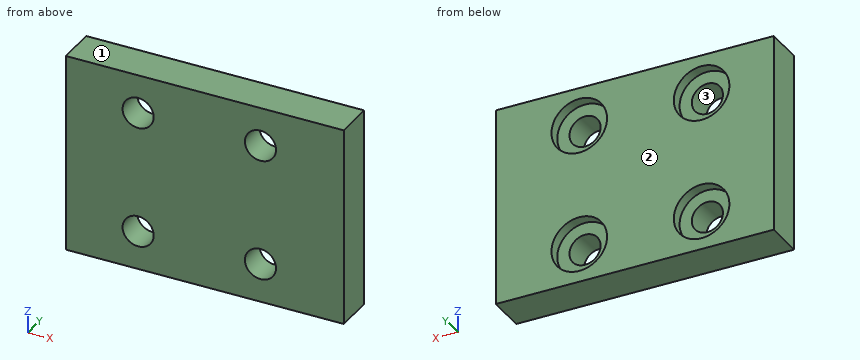
```python
from build123d import *

# Parameters (mm, degrees)
SKETCH1_W           = 50
SKETCH1_H           = 36
BOSS_EXTRUDE1_DEPTH = 7
SKETCH2_R           = 2.8
CUT_EXTRUDE1_DEPTH  = 63.008063992
SKETCH3_R           = 5
CUT_EXTRUDE2_DEPTH  = 2


with BuildPart() as part:
    # Sketch1 → Boss-Extrude1 (new body)
    with BuildSketch(Plane(origin=(0, 0, 0), x_dir=(1, 0, 0), z_dir=(0, 1, 0))):
        with Locations((25, 18)):
            Rectangle(SKETCH1_W, SKETCH1_H)
    extrude(amount=BOSS_EXTRUDE1_DEPTH)

    # Sketch2 → Cut-Extrude1 (cut, through all)
    with BuildSketch(Plane(origin=(0, 7, 0), x_dir=(1, 0, 0), z_dir=(0, 1, 0))):
        with Locations(Location((13, 29, 0), (0, 0, 270))):
            Circle(SKETCH2_R)
        with Locations(Location((13, 7, 0), (0, 0, 90))):
            Circle(SKETCH2_R)
        with Locations(Location((35, 29, 0), (0, 0, 270))):
            Circle(SKETCH2_R)
        with Locations(Location((35, 7, 0), (0, 0, 270))):
            Circle(SKETCH2_R)
    extrude(amount=-CUT_EXTRUDE1_DEPTH, mode=Mode.SUBTRACT)

    # Sketch3 → Cut-Extrude2 (cut)
    with BuildSketch(Plane(origin=(0, 7, 0), x_dir=(1, 0, 0), z_dir=(0, 1, 0))):
        with Locations(Location((13, 29, 0), (0, 0, 270))):
            Circle(SKETCH3_R)
        with Locations(Location((13, 7, 0), (0, 0, 270))):
            Circle(SKETCH3_R)
        with Locations(Location((35, 29, 0), (0, 0, 270))):
            Circle(SKETCH3_R)
        with Locations(Location((35, 7, 0), (0, 0, 270))):
            Circle(SKETCH3_R)
    extrude(amount=-CUT_EXTRUDE2_DEPTH, mode=Mode.SUBTRACT)


solid = part.part
```
Check sheet for the modelled part. Datum: model origin and axes. Units: mm. Face numbers are marked on the shaded views. Round coordinates to 2 decimals unless told otherwise and drop trailing zeros. Loops run counter-clockwise (first coordinate to the right, second up) from the corner with the lowest first, then second, coordinate; pieces in that order, holes last. Notation, with made-up numbers: (28, 11.5) -> (42, 11.5) arc R25 ccw to (42, 45.5) -> close; hole circle Ø9 at (-20, 65). An arc over 180 degrees is marked (long way). Answer in a Markdown table with one row per item.
Q1. Sectioned sample at D-D on y = 5.5. Enter the section's corners in (x, z), then the cut area to 3 significant figures.
Data:
| item | result |
|---|---|
| outline | (0, -36) -> (50, -36) -> (50, 0) -> (0, 0) -> close; hole circle Ø10 at (13, -29); hole circle Ø10 at (13, -7); hole circle Ø10 at (35, -29); hole circle Ø10 at (35, -7) |
| area | 1,490 mm^2 |
Q2. Thickness scan on L1, parallel to X at y = 6.3, z = -29; L2, parallel to X at y = 1.8, z = -7; L3, parallel to Y at x = 10.5, z = -5. Record the ranges inside material, lowest first.
Data:
| item | result |
|---|---|
| L1 | x = 0 to 8, 18 to 30, 40 to 50 |
| L2 | x = 0 to 10.2, 15.8 to 32.2, 37.8 to 50 |
| L3 | y = 0 to 5 |
Q3. Sectioned sample at A-A on x = 13. Enter the section's corners in (y, z), then the cut area to 3 significant figures.
Data:
| item | result |
|---|---|
| outline | (0, -36) -> (7, -36) -> (7, -34) -> (5, -34) -> (5, -31.8) -> (0, -31.8) -> close; (0, -26.2) -> (5, -26.2) -> (5, -24) -> (7, -24) -> (7, -12) -> (5, -12) -> (5, -9.8) -> (0, -9.8) -> close; (0, -4.2) -> (5, -4.2) -> (5, -2) -> (7, -2) -> (7, 0) -> (0, 0) -> close |
| area | 156 mm^2 |
Q4. Sectioned sample at B-B on y = 2.25. Enter the section's corners in (x, z), then the cut area to 3 significant figures.
Data:
| item | result |
|---|---|
| outline | (0, -36) -> (50, -36) -> (50, 0) -> (0, 0) -> close; hole circle Ø5.6 at (13, -29); hole circle Ø5.6 at (13, -7); hole circle Ø5.6 at (35, -29); hole circle Ø5.6 at (35, -7) |
| area | 1,700 mm^2 |
Q5. Sectioned sample at C-C on z = -29. Enter the section's corners in (x, y).
Data:
| item | result |
|---|---|
| outline | (0, 0) -> (10.2, 0) -> (10.2, 5) -> (8, 5) -> (8, 7) -> (0, 7) -> close; (15.8, 0) -> (32.2, 0) -> (32.2, 5) -> (30, 5) -> (30, 7) -> (18, 7) -> (18, 5) -> (15.8, 5) -> close; (37.8, 0) -> (50, 0) -> (50, 7) -> (40, 7) -> (40, 5) -> (37.8, 5) -> close |
Q6. Release check for a two-part mould opening along Z. For the marked faces 1, 2 and 3 record: released by +Z, released by -Z, zero draft, split by the parting line, or undercut.
Data:
| item | result |
|---|---|
| face 1 | released by +Z |
| face 2 | zero draft |
| face 3 | undercut |
Q7. Go/stop test with flat-tipped pins: P1, Ø9, axis at x = 13, z = -29, coming from the +Y side; P2, Ø16, axis at x = 35, z = -29, coming from the +Y side; P3, Ø3, axis at x = 12.5, z = -8, coming from the +Y side. Record where each tip stops, or that it passes through.
Data:
| item | result |
|---|---|
| P1 | stops at y = 5 |
| P2 | stops at y = 7 |
| P3 | passes through |
